Source: CAD feature listing. Evaluate the final solid. Frame: model axes, mm. A direction names the side the tool comes from. Coordinates: 2 decimals unless noted, no trailing zeros. Order: outer loops, then holes, each group sorted by start corner. A loop starts at its lowest first (then second) coordinate and runs counter-clockwise, first axis right, second up.
Item 1: Ray query, line 1 (Z direction, x = -4, y = 3.25); line 2 (Y direction, x = 0, z = 6.5); line 3 (Z direction, x = 3, y = -2.5). Return the intervals inside material, ascending.
Item 2: Mould query, pull axis Z, two halves, no side actions, for faces 1 (the flat face through (3, 3, 7.331)), 2 (the conical face through (3.2, -5.49, 10.67)), 3 (the flat face through (5.22, -2.96, 9.01)). Classes: released by +Z, released by -Z, zero draft, split by the parting line, or undercut.
Item 3: Section C-C on z = 5.75. Return the cut outline in (x, y).
Item 4: Reachability of faces 4 (the cylindrical face through (4.64, 1.46, 0.07)), 5 (the cylindrical face through (-0.84, 3.77, 6.79)), 6 (the flat face through (-5.22, 2.96, 9.01)) from +Z, -Z, +X, -X, +Y, -Y: full face, straight path, thin tool, end or side. Return the list, or none.
Item 5: Section A-A on x = 0. Return the cut outline in (y, z).
Item 6: Section B-B on z = -2.75. Return the cut outline in (x, y), then the cut area to 3 significant figures.
Item 7: Contact query for flat-ended pins moving along their axis: P1, Ø1, axis at x = -0.5, z = 6.5, coming from the -Y side; P2, Ø3, axis at x = -4, z = 2, coming from the -Y side; P3, Ø1.5, axis at y = 3.5, z = 8, coming from the +X side. Output: stop coordinate, or through.
Autodesk Inventor part; units mm, degrees
ref_plane "YZ Plane" through (0, 0, 0) normal (1, 0, 0) x (0, 1, 0)
ref_plane "XZ Plane" through (0, 0, 0) normal (0, 1, 0) x (-1, 0, 0)
ref_plane "XY Plane" through (0, 0, 0) normal (0, 0, 1) x (1, 0, 0)
sketch "Szkic7" plane through (0, 0, 0) normal (0, 0, 1) x (1, 0, 0)
  circle A0 centre (0, 0) radius 4.864
  dimension "d35" = 9.728
extrude "Wyciągnięcie proste2" add sketch "Szkic7" along normal mid plane 12.5375
chamfer "Faza2" distance 1 angle 45 1 edges at (-4.864, 0, 6.2688)
sketch "Szkic9" plane through (0, 0, 6.2688) normal (0, 0, 1) x (1, 0, 0)
  circle A0 centre (0, 0) radius 3.864
extrude "Wyciągnięcie proste3" add sketch "Szkic9" along normal blind 1.0625
sketch "Szkic10" plane through (0, 0, 7.3313) normal (0, 0, 1) x (1, 0, 0)
  line L0 (-3.4641, 6) -> (3.4641, 6)
  line L1 (3.4641, 6) -> (6.9282, 0)
  line L2 (6.9282, 0) -> (3.4641, -6)
  line L3 (3.4641, -6) -> (-3.4641, -6)
  line L4 (-3.4641, -6) -> (-6.9282, 0)
  line L5 (-6.9282, 0) -> (-3.4641, 6)
  line L6 (0, 8.4) -> (0, -8.4) construction
  line L7 (-9.6995, 0) -> (9.6995, 0) construction
  point P0 (0, 0)
  point P1 (0, 0)
  point P2 (0, 6)
  dimension "d44" = 12
extrude "Wyciągnięcie proste4" add sketch "Szkic10" along normal blind 3.4
sketch "Szkic12" plane through (0, 0, 0) normal (0, 1, 0) x (-1, 0, 0)
  line L0 (0, -2.1463) -> (0, 12.8775) construction
  line L1 (-3.4641, 7.3313) -> (-3.4641, 10.7313) construction
  line L2 (-6.9282, 10.7313) -> (-3.4641, 10.7313) construction
  line L3 (-6.9282, 7.3313) -> (-6.9282, 10.7313)
  line L4 (-6.9282, 10.5169) -> (-6.1282, 10.7313)
  line L5 (-6.9282, 10.7313) -> (-3.4641, 10.7313)
  line L6 (-6.9282, 7.3313) -> (-3.4641, 7.3313)
  point P0 (0, 0)
  dimension "d50" = 15
  dimension "d51" = 0.8
revolve "Obrót2" cut sketch "Szkic12" angle 360 about axis through (0, 0, -10) along (0, 0, 1)
thread "Gwint3"
chamfer "Faza3" distance 1 angle 45 1 edges at (-4.864, 0, -6.2688)
equation "\"d35\" = OD"
equation "\"d36\" = 0.7375 * L"
equation "\"d42\" = 0.0625 * L"
equation "\"d44\" = SW"
equation "\"d45\" = 0.2 * L"
equation "\"d51\" = 0.0666667 * SW"
equation "\"SzerokośćGięciaPodcięcia\" = Grubość"
equation "\"RozmiarPodcięciaNarożnika\" = 4 * Grubość"
equation "\"PromieńPrzejścia\" = PromieńGięcia"
equation "\"Rozmiar_promienia_Jacobiego\" = PromieńGięcia"
equation "\"Wielk_odstępu\" = Grubość"
equation "\"d2\" = PromieńGięcia"
equation "\"d23\" = PromieńGięcia"
equation "\"OD\" = 9.728"
equation "\"SW\" = 12"
equation "\"L\" = 17"
properties part number "Korek sześciokątny BSP 1/8'' L=17" material "304"
Answer list:
1. line 1: z = 7.33 to 10.73
1. line 2: y = -3.86 to 3.86
1. line 3: z = -6.23 to 6.23, 7.33 to 10.73
2. face 1: undercut
2. face 2: released by +Z
2. face 3: zero draft
3. outline: circle Ø8.77 at (0, 0)
4. face 4: -Z
4. face 5: none
4. face 6: +Z, -Z, -X, +Y
5. outline: (-6, 7.33) - (-3.86, 7.33) - (-3.86, 6.27) - (-4.86, 5.27) - (-4.86, -5.27) - (-3.86, -6.27) - (3.86, -6.27) - (4.86, -5.27) - (4.86, 5.27) - (3.86, 6.27) - (3.86, 7.33) - (6, 7.33) - (6, 10.73) - (-6, 10.73) - close
6. outline: circle Ø9.73 at (0, 0)
6. area: 74.3 mm2
7. P1: stops at y = -4.11
7. P2: stops at y = -4.17
7. P3: stops at x = 5.34
